The drawing under review shows one solid part. Ordinate dimensions are in mm from its lowest x, y, z. Coordinates: 2 decimals unless noted, no trailing zeros. Write each loop counter-clockwise with the first axis right and the second up, starting at its lowest first coordinate (ties: lowest second). Pieces come first, ordered by that corner, then holes.
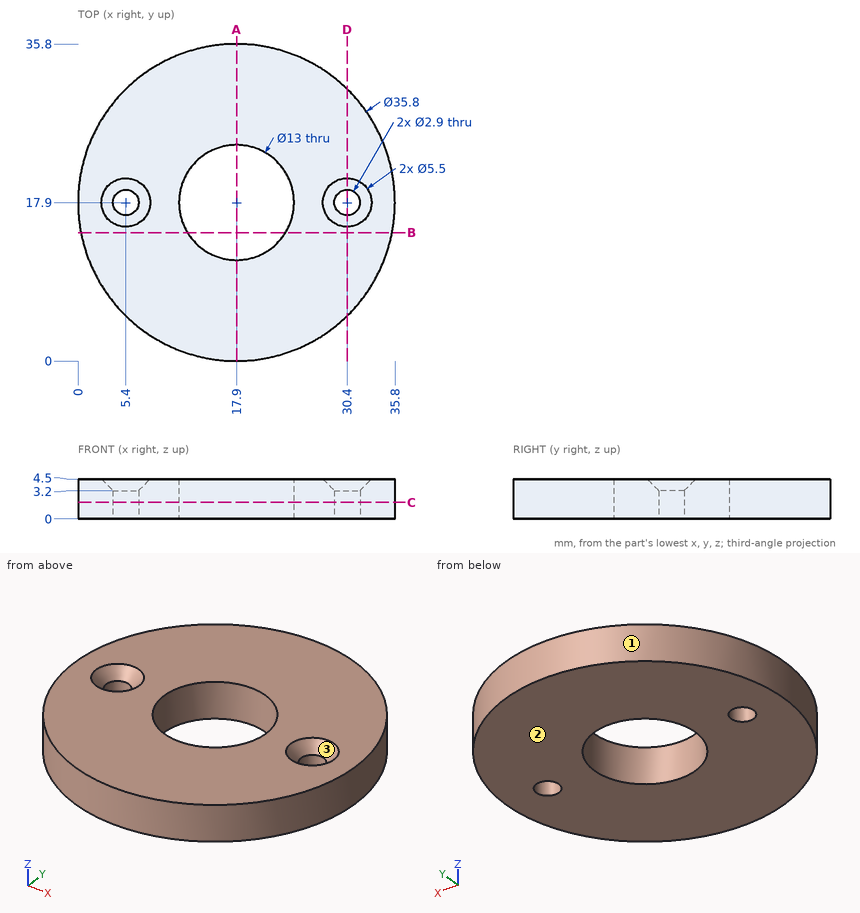
Q1. For probe 1 along X at (y, z) = (13, 1.8); probe 2 along X at (y, z) = (15, 3.55); probe 3 along Y at (x, z) = (30.4, 1.65), list the stretches that pass through material, from the lowest coordinate up.
Ans:
probe 1: x = 0.68 to 13.63, 22.17 to 35.12
probe 2: x = 0.24 to 12.08, 23.72 to 35.56
probe 3: y = 5.09 to 16.45, 19.35 to 30.71
Q2. Add section B-B (y = 14.5). State the section outline as (x, z) points, then the cut area to 3 significant figures.
Ans:
outline: (0.33, 0) - (12.36, 0) - (12.36, 4.5) - (0.33, 4.5) - close; (23.44, 0) - (35.47, 0) - (35.47, 4.5) - (23.44, 4.5) - close
area: 108 mm2
Q3. Add section C-C (z = 1.85). State the section outline as (x, y) points, then the cut area to 3 significant figures.
Ans:
outline: circle Ø35.8 at (17.9, 17.9); hole circle Ø2.9 at (5.4, 17.9); hole circle Ø13 at (17.9, 17.9); hole circle Ø2.9 at (30.4, 17.9)
area: 861 mm2
Q4. Add section A-A (x = 17.9). State the section outline as (y, z) points, then the cut area to 3 significant figures.
Ans:
outline: (0, 0) - (11.4, 0) - (11.4, 4.5) - (0, 4.5) - close; (24.4, 0) - (35.8, 0) - (35.8, 4.5) - (24.4, 4.5) - close
area: 103 mm2
Q5. Draft analysis for pull direction X (two halves, no side actions). For the marked faces 1, 2 and 3, state which applies: +X half, -X half, draft (parallel to the pull), parting line (faces both ways), or undercut.
Ans:
face 1: parting line
face 2: draft
face 3: undercut
Q6. Add section D-D (x = 30.4). State the section outline as (y, z) points, then the cut area to 3 significant figures.
Ans:
outline: (5.09, 0) - (16.45, 0) - (16.45, 3.2) - (15.15, 4.5) - (5.09, 4.5) - close; (19.35, 0) - (30.71, 0) - (30.71, 4.5) - (20.65, 4.5) - (19.35, 3.2) - close
area: 101 mm2
Q7. Clearance check with flat-ended pins moving along their axes: pin 1 Ø1 at (x, z) = (11, 2.5) entering from +Y; pin 2 Ø4.5 at (x, y) = (5.4, 17.9) entering from +Z; pin 3 Ø2.5 at (x, y) = (30.4, 17.9) entering from +Z; pin 4 Ø1.5 at (x, z) = (32, 4) entering from +Y. State where each tip first meets the part, or that it passes through.
Ans:
pin 1: stops at y = 34.62
pin 2: stops at z = 4
pin 3: passes through
pin 4: stops at y = 29.82
